Can you work these out from the drawing? Everything is in mm from the part's minimum corner. A direction names the side the tool comes from. Round coordinates to 2 decimals unless told otherwise and drop trailing zeros. Write each loop counter-clockwise with the first axis right and the second up, starting at its lowest first coordinate (ties: lowest second). Pieces come first, ordered by that corner, then holes. Notation, with made-up numbers: (29.25, 70) -> (71.25, 70) arc R19 ccw to (71.25, 99) -> close; hole circle Ø6 at (57, 4). An arc over 180 degrees is marked (long way). Answer as CSV lines item,"result".
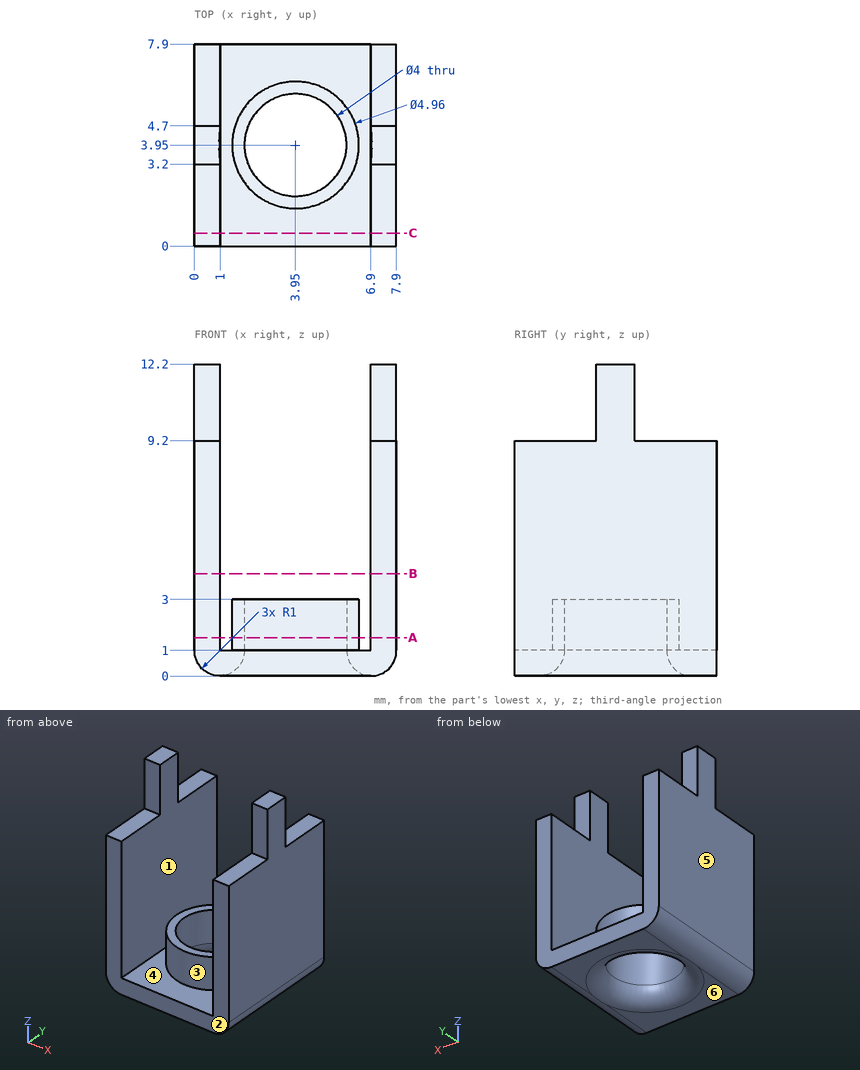
Item 1: Will these pins go through, and if not, where does the flat tip stop? pin 1 (3 mm diameter, centred on x = 4.5, y = 4.5, fed in from +Z); pin 2 (0.8 mm diameter, centred on x = 0.5, y = 2, fed in from +Z); pin 3 (0.8 mm diameter, centred on x = 7.5, z = 10.5, fed in from -Y).
Results found:
pin 1,"stops at z = 3"
pin 2,"stops at z = 9.2"
pin 3,"stops at y = 3.2"
Item 2: For the marked faces 1, 2 and 3, which set-ups out of +Z, -Z, +X, -X, +Y, -Y let a thin tool reach every point of the face, with its end or its side?
Results found:
face 1,"+Z, +Y, -Y"
face 2,"+Z, -Z, +X, -X, -Y"
face 3,"+Z"
Item 3: I need wall thicknesses on L1, parallel to X at y = 1, z = 1.75; L2, parallel to X at y = 3.5, z = 2.25; L3, parallel to Y at x = 3.95, z = 2.1. Which ranges of each line are inside material? Lowest first, please.
Results found:
L1,"x = 0 to 1, 6.9 to 7.9"
L2,"x = 0 to 1, 1.51 to 2, 5.9 to 6.39, 6.9 to 7.9"
L3,"y = 1.47 to 1.95, 5.95 to 6.43"
Item 4: Suppose I cut it at C-C, the plane y = 0.5. List the corners of the cut face in (x, z) for me.
Results found:
outline,"(0, 1) arc R1 ccw to (1, 0) -> (6.9, 0) arc R1 ccw to (7.9, 1) -> (7.9, 9.2) -> (6.9, 9.2) -> (6.9, 1) -> (1, 1) -> (1, 9.2) -> (0, 9.2) -> close"
Item 5: If we mould it in two halves opening along X, with no side actions, what happens to the marked faces 4, 5 and 6? For each: pulls with the +X half, pulls with the -X half, needs draft (parallel to the pull), parting line crosses it, or undercut.
Results found:
face 4,"undercut"
face 5,"pulls with the -X half"
face 6,"needs draft"
Item 6: Suppose I cut it at A-A, the plane z = 1.5. List the corners of the cut face in (x, y) for me.
Results found:
outline,"(0, 0) -> (1, 0) -> (1, 7.9) -> (0, 7.9) -> close; circle Ø4.96 at (3.95, 3.95); (6.9, 0) -> (7.9, 0) -> (7.9, 7.9) -> (6.9, 7.9) -> close; hole circle Ø4 at (3.95, 3.95)"
Item 7: Suppose I cut it at B-B, the plane z = 4. List the corners of the cut face in (x, y) for me.
Results found:
outline,"(0, 0) -> (1, 0) -> (1, 7.9) -> (0, 7.9) -> close; (6.9, 0) -> (7.9, 0) -> (7.9, 7.9) -> (6.9, 7.9) -> close"
